```python
from build123d import *

# Parameters (mm, degrees)
F1_DEPTH = 63.5
F2_DEPTH = 25.4
F3_DEPTH = 7.9375
F5_R     = 6.35


with BuildPart() as f1:
    # F0 (on Front) → F1 (new body, symmetric)
    with BuildSketch(Plane.XZ):
        Polygon((22.225, 9.525), (-41.275, 9.525), (-41.275, -9.525), (41.275, -9.525), (41.275, 9.525), align=None)
    extrude(amount=F1_DEPTH, both=True)

    # F0 (on Front) → F2 (join, symmetric)
    with BuildSketch(Plane.XZ):
        with BuildLine():
            Line((22.225, 30.8886063695), (22.225, 9.525))
            Line((22.225, 9.525), (41.275, 9.525))
            Line((41.275, 9.525), (41.275, 30.8886063695))
            ThreePointArc((41.275, 30.8886063695), (45.9246798487, 42.1139265208), (57.15, 46.7636063695))
            Line((57.15, 46.7636063695), (58.8163197305, 46.7636063695))
            Line((58.8163197305, 46.7636063695), (58.8163197305, 65.8136063695))
            Line((58.8163197305, 65.8136063695), (57.15, 65.8136063695))
            add(Edge.make_bspline(
                [(52.0489083349, 65.4390693016), (53.7508813718, 65.5794651146), (55.4520089295, 65.7039665401), (57.15, 65.8136063695)],
                knots=[109.0031117585, 109.0031117585, 109.0031117585, 109.0031117585, 113.3838076271, 113.3838076271, 113.3838076271, 113.3838076271], degree=3))
            ThreePointArc((52.0489083349, 65.4390693016), (30.7122310756, 53.7096492751), (22.225, 30.8886063695))
        make_face()
        Polygon((79.6208217113, 65.8136063695), (58.8163197305, 65.8136063695), (58.8163197305, 46.7636063695), (58.8163197305, 37.2386063695), (79.3484657375, 37.2386063695), align=None)
    extrude(amount=F2_DEPTH, both=True)

    # F0 (on Front) → F3 (join, symmetric)
    with BuildSketch(Plane.XZ):
        with BuildLine():
            add(Edge.make_bspline(
                [(-41.275, 9.525), (-33.1736003349, 48.6113302876), (9.6993906508, 61.9456561664), (52.0489083349, 65.4390693016)],
                knots=[0, 0, 0, 0, 109.0031117585, 109.0031117585, 109.0031117585, 109.0031117585], degree=3))
            Line((-41.275, 9.525), (22.225, 9.525))
            Line((22.225, 9.525), (22.225, 30.8886063695))
            ThreePointArc((22.225, 30.8886063695), (30.7122310756, 53.7096492751), (52.0489083349, 65.4390693016))
        make_face()
    extrude(amount=F3_DEPTH, both=True)

    # F0 (on Front) → F4 (revolve)
    with BuildSketch(Plane.XZ):
        Polygon((109.6163197305, 65.8136063695), (79.6208217113, 65.8136063695), (79.3484657375, 37.2386063695), (109.6163197305, 37.2386063695), align=None)
    revolve(axis=Axis((79.4846437244, 0, 51.5261063695), (0.0095308348, 0, 0.9999545806)))

    # F5
    f5_edges = [f1.edges().sort_by_distance(p)[0] for p in [
        (-41.275, -63.5, 0),
        (41.275, -63.5, 0),
        (41.275, 63.5, 0),
        (-41.275, 63.5, 0),
    ]]
    fillet(f5_edges, radius=F5_R)


solid = f1.part
```
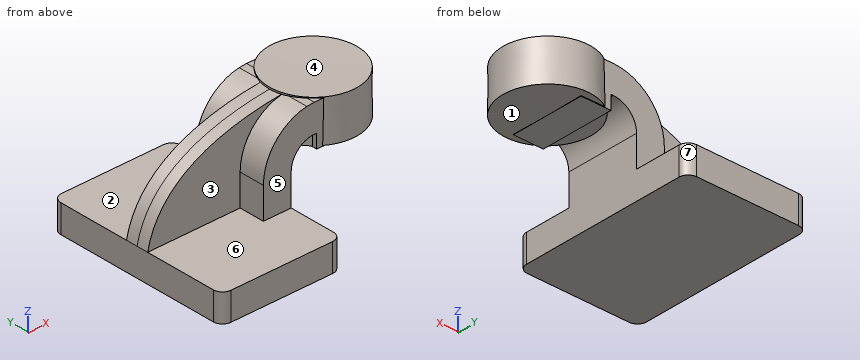
Can you work these out from the model? Positions are in its coordinate system, mm. Face numbers are marked on the shaded views. A direction names the side the tool comes from. Round coordinates to 2 decimals unless told otherwise and drop trailing zeros. Loops run counter-clockwise (first coordinate to the right, second up) from the corner with the lowest first, then second, coordinate; pieces in that order, holes last. Notation, with made-up numbers: M 23,-4 L 50,-4 A31 cw 50,33 Z; hole C 73.5,-7 d7. An arc over 180 degrees is marked long. Answer in a Markdown table with one row per item.
1. On a 3-axis mill with a long thin cutter (end or side, diameter ignored), from which of +Z, -Z, +X, -X, +Y, -Y can I reach the whole of each face in a straight line? I mean the marked faces 1, 2 and 3. Say none if no direction works.
Established:
| item | result |
|---|---|
| face 1 | -Z |
| face 2 | +Z, -X, +Y |
| face 3 | +Z, -X, -Y |
2. Thinking about a two-plate mould opening in Y: for the marked faces 4, 5, 6 and 7, which applies, pulls with the +Y half, pulls with the -Y half, needs draft (parallel to the pull), parting line crosses it, or undercut?
Established:
| item | result |
|---|---|
| face 4 | undercut |
| face 5 | pulls with the -Y half |
| face 6 | needs draft |
| face 7 | pulls with the +Y half |
3. I'm going to push flat-ended pins straight in: pin 1 Ø4 at (x, z) = (-10, 20) entering from -Y; pin 2 Ø4.5 at (x, y) = (62, -22) entering from +Z; pin 3 Ø3 at (y, z) = (13, 57.5) entering from +X; pin 4 Ø14 at (y, z) = (-15, 15.5) entering from -X (3 decimals). Where does each tip first touch, or does it pass through?
Established:
| item | result |
|---|---|
| pin 1 | y = -7.94 |
| pin 2 | z = 66.29 |
| pin 3 | x = 107.33 |
| pin 4 | x = -41.275 |
4. If we section it at A-A, the plane y = 48: Please give me the cut outline in (x, z) (3 decimals), plus the area to 3 significant figures.
Established:
| item | result |
|---|---|
| outline | M -41.275,-9.525 L 41.275,-9.525 L 41.275,9.525 L -41.275,9.525 Z |
| area | 1,570 mm² |
5. Please list where these lines run through material, in increasing order: line 1 (Y direction, x = 35, z = 35); line 2 (Z direction, x = 32, y = -47) (3 decimals); line 3 (X direction, y = 38.5, z = 3.5) (3 decimals). Write a range as from..to.
Established:
| item | result |
|---|---|
| line 1 | -25.4..25.4 |
| line 2 | -9.525..9.525 |
| line 3 | -41.275..41.275 |
